Input: part model. Units: mm. Frame: model coordinates. Face numbers are marked on the shaded views. A direction names the side the tool comes from. Give positions to 0.01 mm unless a question says otherwise; leave off trailing zeros. Order: outer loops, then holes, each group sorted by start corner. A loop starts at its lowest first (then second) coordinate and runs counter-clockwise, first axis right, second up. Notation, with made-up numbers: (-35, 73.5) - (-12, 73.5) arc R12 ccw to (-12, 87.5) - close; hole circle Ø1 at (34, -25). An arc over 180 degrees is marked (long way). Use a Markdown table: item, result.
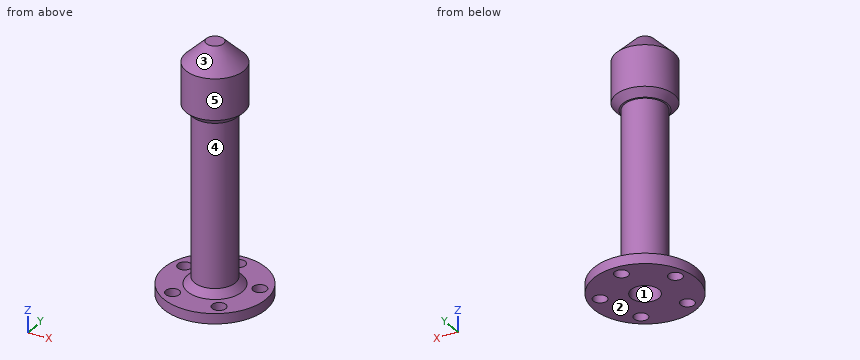
from build123d import *

# Parameters (mm, degrees)
SKETCH1_R           = 15
BOSS_EXTRUDE1_DEPTH = 3
SKETCH2_R           = 2
CUT_EXTRUDE1_DEPTH  = 3
SKETCH3_R           = 6
BOSS_EXTRUDE5_DEPTH = 50
CHAMFER1_SIZE       = 2
SKETCH5_R           = 8.5
BOSS_EXTRUDE6_DEPTH = 20
CHAMFER2_SIZE       = 6
CHAMFER3_SIZE       = 2
SKETCH6_R           = 4.1
CUT_EXTRUDE2_DEPTH  = 60


with BuildPart() as part:
    # Sketch1 → Boss-Extrude1 (new body)
    with BuildSketch(Plane.XY):
        Circle(SKETCH1_R)
    extrude(amount=BOSS_EXTRUDE1_DEPTH)

    # Sketch2 → Cut-Extrude1 (cut)
    with BuildSketch(Plane.XY.offset(3)):
        with Locations((0, 11.5)):
            Circle(SKETCH2_R)
        with Locations((10.937149937, 3.553695435)):
            Circle(SKETCH2_R)
        with Locations((6.759530401, -9.303695435)):
            Circle(SKETCH2_R)
        with Locations((-6.759530401, -9.303695435)):
            Circle(SKETCH2_R)
        with Locations((-10.937149937, 3.553695435)):
            Circle(SKETCH2_R)
    extrude(amount=-CUT_EXTRUDE1_DEPTH, mode=Mode.SUBTRACT)

    # Sketch3 → Boss-Extrude5 (add)
    with BuildSketch(Plane.XY.offset(3)):
        Circle(SKETCH3_R)
    extrude(amount=BOSS_EXTRUDE5_DEPTH)

    # Chamfer1
    chamfer1_edges = [part.edges().sort_by_distance(p)[0] for p in [
        (-6, 0, 3),
    ]]
    chamfer(chamfer1_edges, length=CHAMFER1_SIZE)

    # Sketch5 → Boss-Extrude6 (add)
    with BuildSketch(Plane.XY.offset(53)):
        Circle(SKETCH5_R)
    extrude(amount=BOSS_EXTRUDE6_DEPTH)

    # Chamfer2
    chamfer2_edges = [part.edges().sort_by_distance(p)[0] for p in [
        (-8.5, 0, 73),
    ]]
    chamfer(chamfer2_edges, length=CHAMFER2_SIZE)

    # Chamfer3
    chamfer3_edges = [part.edges().sort_by_distance(p)[0] for p in [
        (-8.5, 0, 53),
    ]]
    chamfer(chamfer3_edges, length=CHAMFER3_SIZE)

    # Sketch6 → Cut-Extrude2 (cut)
    with BuildSketch(Plane(origin=(0, 0, 0), x_dir=(-1, 0, 0), z_dir=(0, 0, -1))):
        Circle(SKETCH6_R)
    extrude(amount=-CUT_EXTRUDE2_DEPTH, mode=Mode.SUBTRACT)


solid = part.part
1. Set-up query: the marked faces 4 and 5. Return all of +Z, -Z, +X, -X, +Y, -Y with unobstructed straight access to the full face (end or side cutting, diameter ignored); none if empty.
Response:
| item | result |
|---|---|
| face 4 | none |
| face 5 | +Z |
2. Section query B-B (y = 0). Return loops of the section in (x, z).
Response:
| item | result |
|---|---|
| outline | (-15, 0) - (-4.1, 0) - (-4.1, 60) - (4.1, 60) - (4.1, 0) - (15, 0) - (15, 3) - (8, 3) - (6, 5) - (6, 53) - (6.5, 53) - (8.5, 55) - (8.5, 67) - (2.5, 73) - (-2.5, 73) - (-8.5, 67) - (-8.5, 55) - (-6.5, 53) - (-6, 53) - (-6, 5) - (-8, 3) - (-15, 3) - close |
3. Pin query (flat end, axial travel): pin 1 (1.5 mm diameter, centred on x = -4.5, y = 5, fed in from +Z); pin 2 (6.5 mm diameter, centred on x = 10.94, y = 3.55, fed in from +Z); pin 3 (6 mm diameter, centred on y = -7.5, z = 36, fed in from -X). Return the tip coordinate at first contact, or that it passes through.
Response:
| item | result |
|---|---|
| pin 1 | stops at z = 69.52 |
| pin 2 | stops at z = 67.25 |
| pin 3 | stops at x = -3.97 |
4. Material intervals for line 1 along Y through (x, z) = (0, 2.1); line 2 along Y through (x, z) = (0, 17.5); line 3 along X through (y, z) = (-0.25, 5), sorted ascending.
Response:
| item | result |
|---|---|
| line 1 | y = -15 to -4.1, 4.1 to 9.5, 13.5 to 15 |
| line 2 | y = -6 to -4.1, 4.1 to 6 |
| line 3 | x = -5.99 to -4.09, 4.09 to 5.99 |
5. Mould query, pull axis X, two halves, no side actions, for the marked faces 1, 2 and 3. Classes: pulls with the +X half, pulls with the -X half, needs draft (parallel to the pull), parting line crosses it, or undercut.
Response:
| item | result |
|---|---|
| face 1 | undercut |
| face 2 | needs draft |
| face 3 | parting line crosses it |
6. Section query A-A (x = 0). Return loops of the section in (y, z).
Response:
| item | result |
|---|---|
| outline | (-15, 0) - (-4.1, 0) - (-4.1, 60) - (4.1, 60) - (4.1, 0) - (9.5, 0) - (9.5, 3) - (8, 3) - (6, 5) - (6, 53) - (6.5, 53) - (8.5, 55) - (8.5, 67) - (2.5, 73) - (-2.5, 73) - (-8.5, 67) - (-8.5, 55) - (-6.5, 53) - (-6, 53) - (-6, 5) - (-8, 3) - (-15, 3) - close; (13.5, 0) - (15, 0) - (15, 3) - (13.5, 3) - close |
7. Section query D-D (z = 57). Return loops of the section in (x, y), then the cut area to 3 significant figures.
Response:
| item | result |
|---|---|
| outline | circle Ø17 at (0, 0); hole circle Ø8.2 at (0, 0) |
| area | 174 mm^2 |
8. Section query C-C (y = 11.5). Return loops of the section in (x, z).
Response:
| item | result |
|---|---|
| outline | (-9.63, 0) - (-2, 0) - (-2, 3) - (-9.63, 3) - close; (2, 0) - (9.63, 0) - (9.63, 3) - (2, 3) - close |
